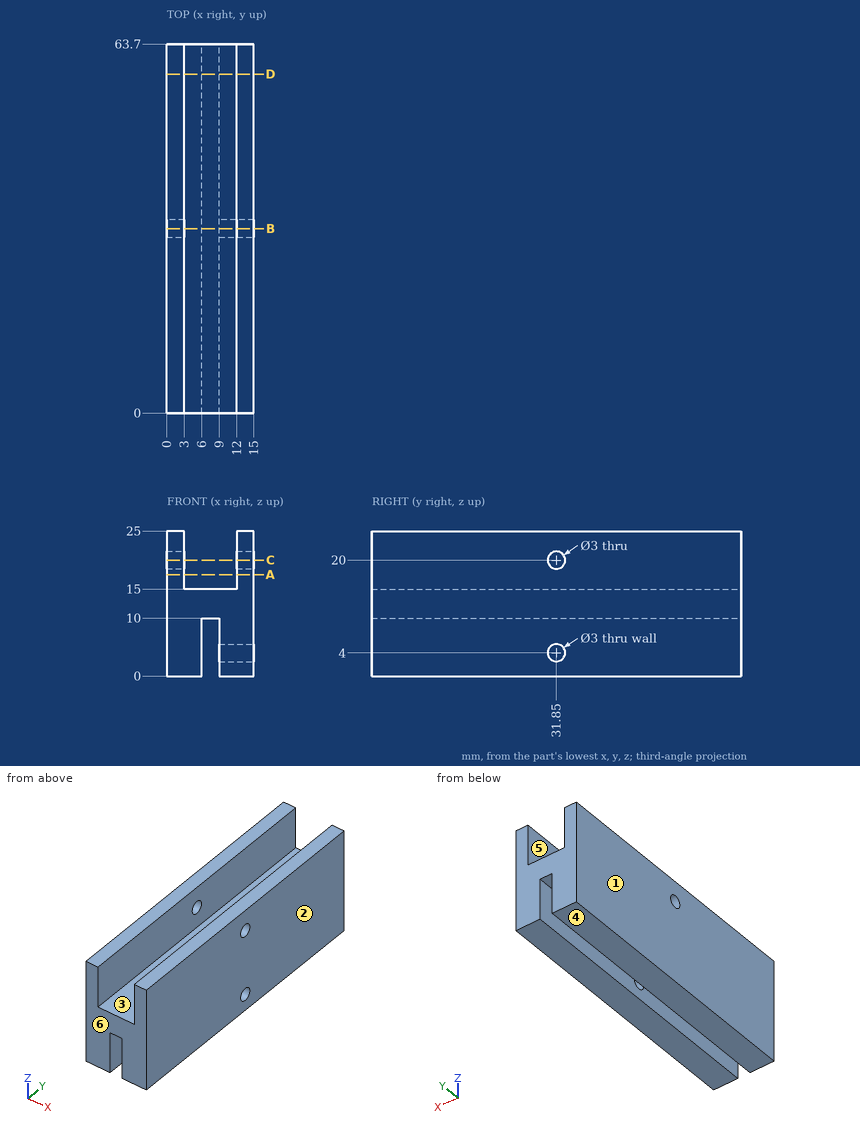
Can you work these out from the drawing? Everything is in mm from the part's minimum corner. A direction names the side the tool comes from. Round coordinates to 2 decimals unless told otherwise and drop trailing zeros. Loops run counter-clockwise (first coordinate to the right, second up) from the corner with the lowest first, then second, coordinate; pieces in that order, holes last. Notation, with made-up numbers: (11.5, 81) - (25.5, 81) arc R16 ccw to (25.5, 104) - close; hole circle Ø7 at (-38, 61). An arc over 180 degrees is marked (long way). Write item = value, one per line. Start each with the question number.
(1) If I drill on probe 1 along Z at (x, y) = (12.7, 31.85); probe 2 along X at (y, z) = (55, 17.5); probe 3 along X at (y, z) = (27, 5.25), over which ranges is the centre line in solid material (lowest first)? Write a range as [from, to].
(2) If we section it at A-A (z = 17.5): Please give me the cut outline in (x, y).
(3) If we mould it in two halves opening along X, with no side actions, what happens to the marked faces 1, 2, 3 and 4? For each: released by +X, released by -X, zero draft, split by the parting line, or undercut.
(4) For the marked faces 5 and 6, which set-ups out of +Z, -Z, +X, -X, +Y, -Y let a thin tool reach every point of the face, with its end or its side?
(5) If we section it at C-C (z = 20): Please give me the cut outline in (x, y).
(6) For P1, Ø1, axis at x = 11, y = 16.5, coming from the -Z side; P2, Ø2.5, axis at y = 31.85, z = 20, coming from the -X side; P3, Ø2.5, axis at x = 7, y = 40.5, coming from the +Z side; P4, Ø2.5, axis at y = 31.85, z = 4, coming from the +X side, each with a flat end and sliding along its axis, tell me the tip position at first contact or that it passes through.
(7) If we section it at D-D (y = 58.5): Please give me the cut outline in (x, z).
(8) If we section it at B-B (y = 31.85): Please give me the cut outline in (x, z), and give its area (3 significant figures).
Ans:
q1.probe_1 = [0, 2.5], [5.5, 18.5], [21.5, 25]
q1.probe_2 = [0, 3], [12, 15]
q1.probe_3 = [0, 6], [9, 15]
q2.outline = (0, 0) - (3, 0) - (3, 63.7) - (0, 63.7) - close; (12, 0) - (15, 0) - (15, 63.7) - (12, 63.7) - close
q3.face_1 = released by -X
q3.face_2 = released by +X
q3.face_3 = undercut
q3.face_4 = zero draft
q4.face_5 = +Z, +Y, -Y
q4.face_6 = +Z, -Z, +X, -X, -Y
q5.outline = (0, 0) - (3, 0) - (3, 30.35) - (0, 30.35) - close; (0, 33.35) - (3, 33.35) - (3, 63.7) - (0, 63.7) - close; (12, 0) - (15, 0) - (15, 30.35) - (12, 30.35) - close; (12, 33.35) - (15, 33.35) - (15, 63.7) - (12, 63.7) - close
q6.P1 = 0
q6.P2 = through
q6.P3 = 15
q6.P4 = 6
q7.outline = (0, 0) - (6, 0) - (6, 10) - (9, 10) - (9, 0) - (15, 0) - (15, 25) - (12, 25) - (12, 15) - (3, 15) - (3, 25) - (0, 25) - close
q8.outline = (0, 0) - (6, 0) - (6, 10) - (9, 10) - (9, 5.5) - (15, 5.5) - (15, 18.5) - (12, 18.5) - (12, 15) - (3, 15) - (3, 18.5) - (0, 18.5) - close; (0, 21.5) - (3, 21.5) - (3, 25) - (0, 25) - close; (9, 0) - (15, 0) - (15, 2.5) - (9, 2.5) - close; (12, 21.5) - (15, 21.5) - (15, 25) - (12, 25) - close
q8.area = 219 mm²
